from build123d import *

# Parameters (mm, degrees)
F0_W     = 609.6
F0_H     = 609.6
F1_DEPTH = 7.9375
F2_R     = 6.35
F3_DEPTH = 12.7
F4_R     = 6.35
F5_DEPTH = 12.7
F6_R     = 6.35
F7_DEPTH = 12.7
F8_R     = 6.35
F9_DEPTH = 12.7


# Not quite as in the source:
# - a length typed as a fraction of an inch, garbled in the dataset ("3 / 203.2 mm" for 3/8 in), is restored


with BuildPart() as f1:
    # F0 (on Top) → F1 (new body, symmetric)
    with BuildSketch(Plane.XY):
        Rectangle(F0_W, F0_H)
    extrude(amount=F1_DEPTH, both=True)

    # F2 (on face) → F3 (join)
    with BuildSketch(Plane.YZ.offset(304.8)):
        Circle(F2_R)
    extrude(amount=F3_DEPTH)

    # F4 (on face) → F5 (cut)
    with BuildSketch(Plane.XZ.offset(304.8)):
        Circle(F4_R)
    extrude(amount=-F5_DEPTH, mode=Mode.SUBTRACT)

    # F6 (on face) → F7 (join)
    with BuildSketch(Plane(origin=(-304.8, 0, 0), x_dir=(0, -1, 0), z_dir=(-1, 0, 0))):
        Circle(F6_R)
    extrude(amount=F7_DEPTH)

    # F8 (on face) → F9 (cut)
    with BuildSketch(Plane(origin=(0, 304.8, 0), x_dir=(-1, 0, 0), z_dir=(0, 1, 0))):
        Circle(F8_R)
    extrude(amount=-F9_DEPTH, mode=Mode.SUBTRACT)


solid = f1.part
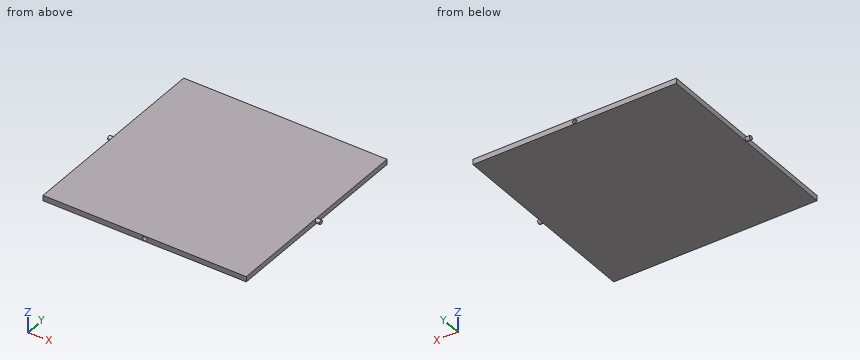
The listing builds one solid part. Answer for the finished solid, in the listing's coordinates (mm). Round coordinates to 2 decimals unless told otherwise and drop trailing zeros. Order: outer loops, then holes, each group sorted by start corner. A loop starts at its lowest first (then second) coordinate and runs counter-clockwise, first axis right, second up. Notation, with made-up numbers: (62.25, 3) -> (66.25, 3) arc R9 cw to (66.25, 14) -> close; hole circle Ø1 at (-2, 54). An arc over 180 degrees is marked (long way). Write each question's results on one line, items separated by ' | '. Start each with the question number.
Q1. Each of these flat-tipped pins is pushed along its axis until it touches: pin 1 (6.5 mm diameter, centred on x = -0.5, z = 2.5, fed in from +Y); pin 2 (1 mm diameter, centred on y = -37.5, z = 1.5, fed in from +X); pin 3 (8 mm diameter, centred on y = -60, z = 2.5, fed in from -X). Where does it stop, or does it pass through?
Q2. Find section A-A (z = 2.5). Determine the outline of the cut face in (x, y).
Q3. Find section B-B (y = -50). Determine the outline of the cut face in (x, z).
Q4. Straight lines are drawn through the part: probe 1 along Z at (x, y) = (0, 297); probe 2 along X at (y, z) = (50, 3.5). For each, find the intervals that lie inside material, in ascending order. Write a range as from..to.
Worked answers:
1) pin 1: stops at y = 292.1 | pin 2: stops at x = 304.8 | pin 3: stops at x = -304.8
2) outline: (-317.5, -5.84) -> (-304.8, -5.84) -> (-304.8, -304.8) -> (-5.84, -304.8) -> (-5.84, -292.1) -> (5.84, -292.1) -> (5.84, -304.8) -> (304.8, -304.8) -> (304.8, -5.84) -> (317.5, -5.84) -> (317.5, 5.84) -> (304.8, 5.84) -> (304.8, 304.8) -> (5.84, 304.8) -> (5.84, 292.1) -> (-5.84, 292.1) -> (-5.84, 304.8) -> (-304.8, 304.8) -> (-304.8, 5.84) -> (-317.5, 5.84) -> close
3) outline: (-304.8, -7.94) -> (304.8, -7.94) -> (304.8, 7.94) -> (-304.8, 7.94) -> close
4) probe 1: z = -7.94..-6.35, 6.35..7.94 | probe 2: x = -304.8..304.8
